Part print with two shaded views. Sizes in mm from the minimum x, y, z corner. A direction names the side the tool comes from. Round coordinates to 2 decimals unless told otherwise and drop trailing zeros. Order: outer loops, then holes, each group sorted by start corner. A loop starts at its lowest first (then second) coordinate and runs counter-clockwise, first axis right, second up. Notation, with made-up numbers: (-1.75, 54) -> (4.25, 54) arc R15 cw to (4.25, 64) -> close; hole circle Ø5 at (68, -28). An arc over 180 degrees is marked (long way). Put each result on its own line as item: value. Start each with the question number.
Q1. Cut at C-C, the plane z = 18. List the corners of the cut face in (x, y), and give its area (3 significant figures).
Q2. Cut at A-A, the plane y = 9. List the corners of the cut face in (x, z), and give its area (3 significant figures).
Q3. Cut at D-D, the plane z = 14. List the corners of the cut face in (x, y), and give its area (3 significant figures).
Q4. Probe L1, parallel to Z at x = 5.75, y = 16; L2, parallel to Z at x = 6, y = 8.75; L3, parallel to Y at x = 7.5, z = 6.5. List the from-to ranges inside material, lowest first.
Q5. Flat gauge pins, fed straight in: P1, Ø3, axis at y = 15.5, z = 13, coming from the -X side; P2, Ø8, axis at x = 7.5, y = 3, coming from the -Z side; P3, Ø5, axis at x = 2.5, z = 9.5, coming from the -Y side. Where does each tip first touch, or does it go through?
Q6. 3-axis set-ups, long thin cutter, end or side, ignore diameter. For the marked faces 1 and 2: which of +Z, -Z, +X, -X, +Y, -Y reach the whole face in a straight line?
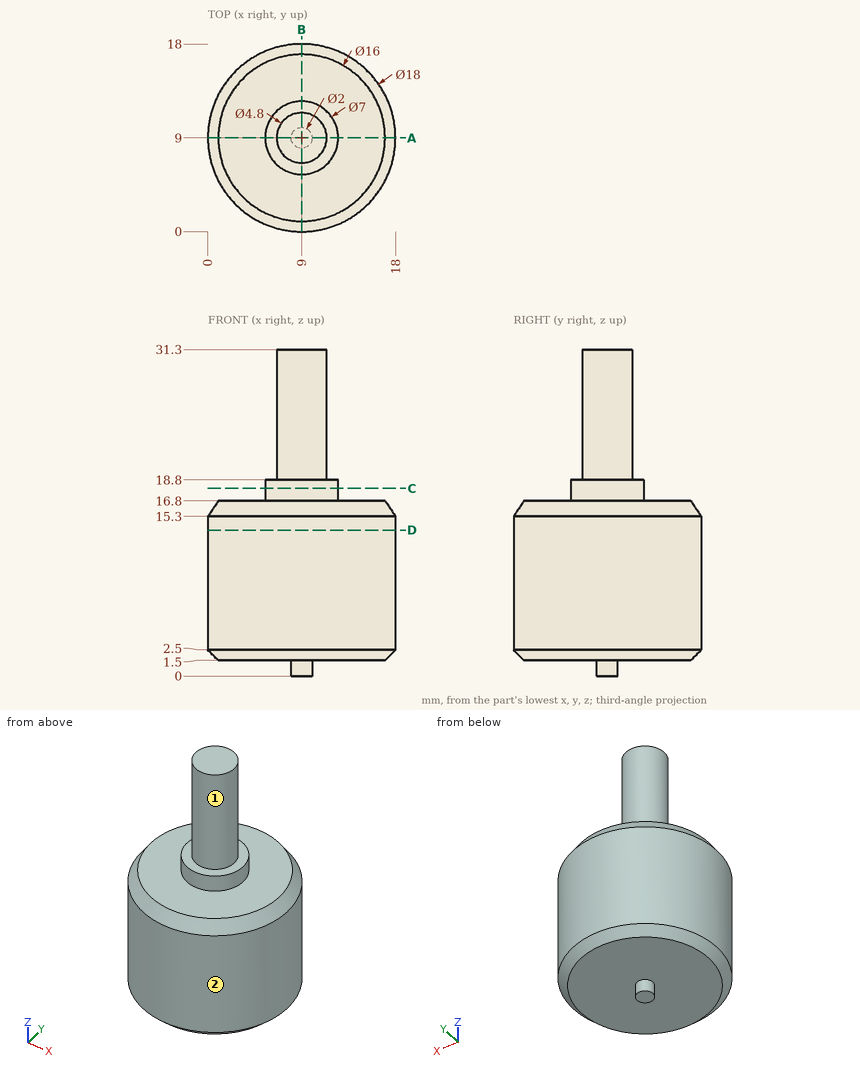
Ans:
1. outline: circle Ø7 at (9, 9)
1. area: 38.5 mm^2
2. outline: (0, 2.5) -> (1, 1.5) -> (8, 1.5) -> (8, 0) -> (10, 0) -> (10, 1.5) -> (17, 1.5) -> (18, 2.5) -> (18, 15.3) -> (17, 16.8) -> (12.5, 16.8) -> (12.5, 18.8) -> (11.4, 18.8) -> (11.4, 31.3) -> (6.6, 31.3) -> (6.6, 18.8) -> (5.5, 18.8) -> (5.5, 16.8) -> (1, 16.8) -> (0, 15.3) -> close
2. area: 350 mm^2
3. outline: circle Ø18 at (9, 9)
3. area: 254 mm^2
4. L1: z = 1.5 to 16.8
4. L2: z = 1.5 to 18.8
4. L3: y = 0.13 to 17.87
5. P1: stops at x = 1.52
5. P2: stops at z = 1.5
5. P3: stops at y = 0.94
6. face 1: +Z
6. face 2: +Z, -Z
